```python
from build123d import *

# Parameters (mm, degrees)
F0_R     = 33.03147
F1_DEPTH = 50.8
F2_R     = 21.247393
F3_DEPTH = 203.2
F4_R     = 5.08
F5_R     = 5.08
F6_R     = 5.08


with BuildPart() as f1:
    # F0 (on Front) → F1 (new body)
    with BuildSketch(Plane.XZ):
        Circle(F0_R)
    extrude(amount=F1_DEPTH)

    # F2 (on Front) → F3 (join)
    with BuildSketch(Plane.XZ):
        Circle(F2_R)
    extrude(amount=F3_DEPTH)

    # F4
    f4_edges = [f1.edges().sort_by_distance(p)[0] for p in [
        (-33.03147, 0, 0),
    ]]
    fillet(f4_edges, radius=F4_R)

    # F5
    f5_edges = [f1.edges().sort_by_distance(p)[0] for p in [
        (-33.03147, -50.8, 0),
    ]]
    fillet(f5_edges, radius=F5_R)

    # F6
    f6_edges = [f1.edges().sort_by_distance(p)[0] for p in [
        (-21.247393, -50.8, 0),
        (-21.247393, -203.2, 0),
    ]]
    fillet(f6_edges, radius=F6_R)


solid = f1.part
```
Model file for the job. Use its own axes, mm. A direction names the side the tool comes from. Round coordinates to 2 decimals unless told otherwise and drop trailing zeros. Write each loop counter-clockwise with the first axis right and the second up, starting at its lowest first coordinate (ties: lowest second). Pieces come first, ordered by that corner, then holes. Notation, with made-up numbers: (82.25, 10.25) - (94.25, 10.25) arc R22 cw to (94.25, 21.25) - close; hole circle Ø1 at (20.5, -10). An arc over 180 degrees is marked (long way). One line per item, written item: value.
(1) Cut at D-D, the plane y = -23. Give the cut face in (x, z), plus the area to 3 significant figures.
Values follow:
outline: circle Ø66.06 at (0, 0)
area: 3,430 mm²
(2) Wall check: probe 1 along Y at (x, z) = (26, 5); probe 2 along Z at (x, y) = (-9, -141); probe 3 along Z at (x, y) = (-17, -168). Give the ranges that are in metal, low to high.
Values follow:
probe 1: y = -50.8 to 0
probe 2: z = -19.25 to 19.25
probe 3: z = -12.75 to 12.75
(3) Cut at A-A, the plane x = 0. Give the cut face in (y, z), plus the area to 3 significant figures.
Values follow:
outline: (-203.2, -16.17) arc R5.08 ccw to (-198.12, -21.25) - (-55.88, -21.25) arc R5.08 cw to (-50.8, -26.33) - (-50.8, -27.95) arc R5.08 ccw to (-45.72, -33.03) - (-5.08, -33.03) arc R5.08 ccw to (0, -27.95) - (0, 27.95) arc R5.08 ccw to (-5.08, 33.03) - (-45.72, 33.03) arc R5.08 ccw to (-50.8, 27.95) - (-50.8, 26.33) arc R5.08 cw to (-55.88, 21.25) - (-198.12, 21.25) arc R5.08 ccw to (-203.2, 16.17) - close
area: 9,810 mm²
(4) Cut at B-B, the plane z = 0. Give the cut face in (x, y), plus the area to 3 significant figures.
Values follow:
outline: (-33.03, -45.72) arc R5.08 ccw to (-27.95, -50.8) - (-26.33, -50.8) arc R5.08 cw to (-21.25, -55.88) - (-21.25, -198.12) arc R5.08 ccw to (-16.17, -203.2) - (16.17, -203.2) arc R5.08 ccw to (21.25, -198.12) - (21.25, -55.88) arc R5.08 cw to (26.33, -50.8) - (27.95, -50.8) arc R5.08 ccw to (33.03, -45.72) - (33.03, -5.08) arc R5.08 ccw to (27.95, 0) - (-27.95, 0) arc R5.08 ccw to (-33.03, -5.08) - close
area: 9,810 mm²
(5) Cut at C-C, the plane y = -154.5. Give the cut face in (x, z).
Values follow:
outline: circle Ø42.49 at (0, 0)
(6) Drop flat-ended pins along their axis: P1, Ø1, axis at x = -23.5, y = -145, coming from the +Z side; P2, Ø12, axis at y = -141, z = -22, coming from the +X side; P3, Ø8, axis at x = -12.5, z = 17.5, coming from the -Y side; P4, Ø5, axis at y = -41.5, z = -8, coming from the +X side. Give the stop position or say it passes through.
Values follow:
P1: passes through
P2: stops at x = 13.98
P3: stops at y = -203.02
P4: stops at x = 32.57
(7) 3-axis set-ups, long thin cutter, end or side, ignore diameter. For faces 1 (the cylindrical face through (31.506, -25.116, 9.922)), 2 (the cylindrical face through (-2.766, -126.004, 21.067)): which of +Z, -Z, +X, -X, +Y, -Y reach the whole face in a straight line?
Values follow:
face 1: +Y, -Y
face 2: -Y
